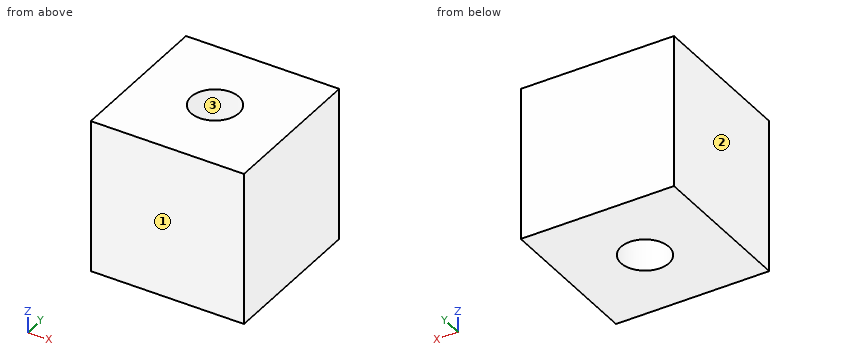
from build123d import *

# Parameters (mm, degrees)
SKETCH1_W           = 48
SKETCH1_H           = 48
BOSS_EXTRUDE1_DEPTH = 48
SKETCH2_R           = 7.5
CUT_EXTRUDE1_DEPTH  = 49


with BuildPart() as part:
    # Sketch1 → Boss-Extrude1 (new body)
    with BuildSketch(Plane(origin=(0, 0, 0), x_dir=(1, 0, 0), z_dir=(0, 1, 0))):
        Rectangle(SKETCH1_W, SKETCH1_H)
    extrude(amount=BOSS_EXTRUDE1_DEPTH)

    # Sketch2 → Cut-Extrude1 (cut, through all)
    with BuildSketch(Plane.XY.offset(24)):
        with Locations((0, 24)):
            Circle(SKETCH2_R)
    extrude(amount=-CUT_EXTRUDE1_DEPTH, mode=Mode.SUBTRACT)


solid = part.part
Could you check a few things on this model? Use its own coordinates, in mm. Face numbers are marked on the shaded views. Round coordinates to 2 decimals unless told otherwise and drop trailing zeros. Write each loop counter-clockwise with the first axis right and the second up, starting at its lowest first coordinate (ties: lowest second). Pieces come first, ordered by that corner, then holes. Notation, with made-up numbers: (83, -15.75) - (101, -15.75) arc R30 ccw to (101, 16.25) - close; hole circle Ø10 at (-18.75, -26). An arc over 180 degrees is marked (long way). Put each result on its own line as item: value. Start each with the question number.
(1) Thinking about a two-plate mould opening in Y: for the marked faces 1, 2 and 3, which applies, released by +Y, released by -Y, zero draft, split by the parting line, or undercut?
(2) I want a section at A-A, the plane x = 0. Please give me the cut outline in (y, z), plus the area to 3 significant figures.
(3) I want a section at B-B, the plane y = 24. Please give me the cut outline in (x, z), plus the area to 3 significant figures.
(4) I want a section at C-C, the plane z = -19. Please give me the cut outline in (x, y), plus the area to 3 significant figures.
(5) I need wall thicknesses on probe 1 along Y at (x, z) = (0, 4); probe 2 along X at (y, z) = (23.5, -11.5); probe 3 along X at (y, z) = (19, 4.5). Which ranges of each line are inside material? Lowest first, please.
Here are the results:
1. face 1: released by -Y
1. face 2: zero draft
1. face 3: undercut
2. outline: (0, -24) - (16.5, -24) - (16.5, 24) - (0, 24) - close; (31.5, -24) - (48, -24) - (48, 24) - (31.5, 24) - close
2. area: 1,580 mm^2
3. outline: (-24, -24) - (-7.5, -24) - (-7.5, 24) - (-24, 24) - close; (7.5, -24) - (24, -24) - (24, 24) - (7.5, 24) - close
3. area: 1,580 mm^2
4. outline: (-24, 0) - (24, 0) - (24, 48) - (-24, 48) - close; hole circle Ø15 at (0, 24)
4. area: 2,130 mm^2
5. probe 1: y = 0 to 16.5, 31.5 to 48
5. probe 2: x = -24 to -7.48, 7.48 to 24
5. probe 3: x = -24 to -5.59, 5.59 to 24
